Part model, mm, in its own coordinate system. Face numbers are marked on the shaded views. A direction names the side the tool comes from. Coordinates: 2 decimals unless noted, no trailing zeros. Loops run counter-clockwise (first coordinate to the right, second up) from the corner with the lowest first, then second, coordinate; pieces in that order, holes last. Notation, with made-up numbers: M 12.25,70 L 21.25,70 A8 ccw 21.25,77 Z; hole C 61.5,-20.75 d4. An arc over 180 degrees is marked long. Answer as a JSON object with one key per item and string values. Group by question number.
1. Drop flat-ended pins along their axis: pin 1 Ø2 at (x, z) = (21, 4.5) entering from -Y; pin 2 Ø4.5 at (x, y) = (22.5, 27) entering from -Z; pin 3 Ø12 at (x, y) = (25, -12.5) entering from -Z; pin 4 Ø4 at (y, z) = (25.59, -25.5) entering from -X (1 decimal). Give the stop position or say it passes through.
2. Drill centre lines: L1, parallel to Z at x = 37, y = -20.5; L2, parallel to Z at x = 38, y = -22; L3, parallel to Z at x = 3, y = 26. Where is each one in solid material? Low to high.
3. Saw through at B-B on x = 26. Count the separate pieces of the cut face and the enclosed holes in it, then the cut area to 3 significant figures.
4. 3-axis set-ups, long thin cutter, end or side, ignore diameter. For the marked faces 5 and 6: which of +Z, -Z, +X, -X, +Y, -Y reach the whole face in a straight line?
5. Saw through at A-A on y = -19. Write the cut outline in (x, z), then the cut area to 3 significant figures.
6. Mould opens along Z. For the marked faces 1, 2, 3 and 4 say: released by +Z, released by -Z, zero draft, split by the parting line, or undercut.
7. Saw through at C-C on z = -18. Write the cut outline in (x, y).
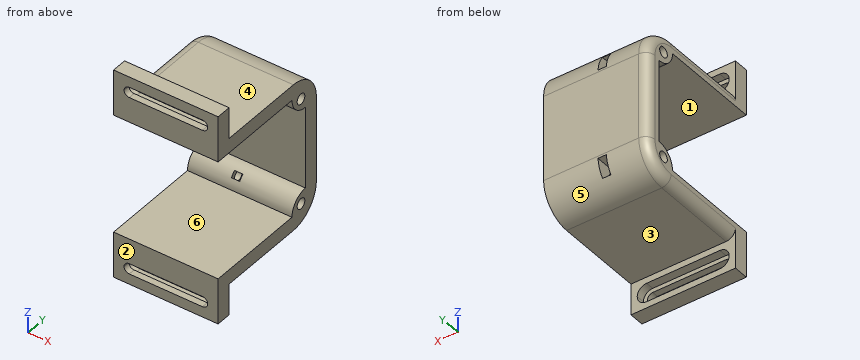
from build123d import *

# Parameters (mm, degrees)
BOSS_EXTRUDE1_DEPTH = 50
SKETCH2_R           = 2.5
CUT_EXTRUDE1_DEPTH  = 50
FILLET1_R           = 15
SKETCH3_W           = 4
SKETCH3_H           = 8
CUT_EXTRUDE2_DEPTH  = 14.54
SKETCH4_W           = 44
SKETCH4_H           = 9
CUT_EXTRUDE3_DEPTH  = 4
SKETCH5_W           = 40
SKETCH5_H           = 5
CUT_EXTRUDE4_DEPTH  = 94.654951818
FILLET2_R           = 2.5
FILLET3_R           = 4.5
FILLET4_R           = 4.5


with BuildPart() as part:
    # Sketch1 → Boss-Extrude1 (new body)
    with BuildSketch(Plane(origin=(0, 0, 0), x_dir=(0, 0, -1), z_dir=(1, 0, 0))):
        with BuildLine():
            Line((35.5, 35.62933491), (-35.5, 35.62933491))
            Line((-35.5, 35.62933491), (-35.5, -21.37066509))
            Line((-35.5, -21.37066509), (-50.5, -21.37066509))
            Line((-50.5, -21.37066509), (-50.5, -28.5))
            Line((-50.5, -28.5), (-28.5, -28.5))
            Line((-28.5, -28.5), (-28.5, 19.7))
            ThreePointArc((-28.5, 19.7), (-22.277460326, 22.277460326), (-19.7, 28.5))
            Line((-19.7, 28.5), (19.7, 28.5))
            ThreePointArc((19.7, 28.5), (22.277460326, 22.277460326), (28.5, 19.7))
            Line((28.5, 19.7), (28.5, -28.5))
            Line((28.5, -28.5), (50.5, -28.5))
            Line((50.5, -28.5), (50.5, -21.37066509))
            Line((50.5, -21.37066509), (35.5, -21.37066509))
            Line((35.5, -21.37066509), (35.5, 35.62933491))
        make_face()
    extrude(amount=BOSS_EXTRUDE1_DEPTH)

    # Sketch2 → Cut-Extrude1 (cut)
    with BuildSketch(Plane.ZY):
        with Locations((-25.5, 25.592902541)):
            Circle(SKETCH2_R)
        with Locations(Location((25.5, 25.592902541, 0), (0, 0, 180))):
            Circle(SKETCH2_R)
    extrude(amount=-CUT_EXTRUDE1_DEPTH, mode=Mode.SUBTRACT)

    # Fillet1
    fillet1_edges = [part.edges().sort_by_distance(p)[0] for p in [
        (25, 35.62933491, 35.5),
        (25, 35.62933491, -35.5),
    ]]
    fillet(fillet1_edges, radius=FILLET1_R)

    # Sketch3 → Cut-Extrude2 (cut)
    with BuildSketch(Plane(origin=(0, 35.62933491, 0), x_dir=(1, 0, 0), z_dir=(0, 1, 0))):
        with Locations((22, 25.5)):
            Rectangle(SKETCH3_W, SKETCH3_H)
        with Locations((22, -25.5)):
            Rectangle(SKETCH3_W, SKETCH3_H)
    extrude(amount=-CUT_EXTRUDE2_DEPTH, mode=Mode.SUBTRACT)

    # Sketch4 → Cut-Extrude3 (cut)
    with BuildSketch(Plane(origin=(0, -21.37066509, 0), x_dir=(1, 0, 0), z_dir=(0, 1, 0))):
        with Locations((25, -43)):
            Rectangle(SKETCH4_W, SKETCH4_H)
        with Locations((25, 43)):
            Rectangle(SKETCH4_W, SKETCH4_H)
    extrude(amount=-CUT_EXTRUDE3_DEPTH, mode=Mode.SUBTRACT)

    # Sketch5 → Cut-Extrude4 (cut, through all)
    with BuildSketch(Plane(origin=(0, -25.37066509, 0), x_dir=(1, 0, 0), z_dir=(0, 1, 0))):
        with Locations((25, -43)):
            Rectangle(SKETCH5_W, SKETCH5_H)
        with Locations((25, 43)):
            Rectangle(SKETCH5_W, SKETCH5_H)
    extrude(amount=-CUT_EXTRUDE4_DEPTH, mode=Mode.SUBTRACT)

    # Fillet2
    fillet2_edges = [part.edges().sort_by_distance(p)[0] for p in [
        (45, -26.935332545, 40.5),
        (45, -26.935332545, 45.5),
        (5, -26.935332545, 45.5),
        (5, -26.935332545, 40.5),
        (5, -26.935332545, -45.5),
        (5, -26.935332545, -40.5),
        (45, -26.935332545, -45.5),
        (45, -26.935332545, -40.5),
    ]]
    fillet(fillet2_edges, radius=FILLET2_R - 0.0001)  # a hair under: the kernel refuses the full size

    # Fillet3
    fillet3_edges = [part.edges().sort_by_distance(p)[0] for p in [
        (3, -23.37066509, 38.5),
        (3, -23.37066509, 47.5),
        (47, -23.37066509, 47.5),
        (47, -23.37066509, 38.5),
        (47, -23.37066509, -47.5),
        (47, -23.37066509, -38.5),
        (3, -23.37066509, -47.5),
        (3, -23.37066509, -38.5),
    ]]
    fillet(fillet3_edges, radius=FILLET3_R - 0.0001)  # a hair under: the kernel refuses the full size

    # Fillet4
    fillet4_edges = [part.edges().sort_by_distance(p)[0] for p in [
        (0, -0.37066509, -35.5),
        (0, -0.37066509, 35.5),
        (0, 35.62933491, 0),
        (0, 31.235936628, -31.106601718),
        (0, 31.235936628, 31.106601718),
    ]]
    fillet(fillet4_edges, radius=FILLET4_R)


solid = part.part
Outcome:
{
 "1": {"pin 1": "stops at y = 28.5", "pin 2": "stops at z = -34.92", "pin 3": "stops at z = -35.5", "pin 4": "passes through"},
 "2": {"L1": "z = -35.5 to -28.5, 28.5 to 35.5", "L2": "z = -50.5 to -47.5, -38.5 to -28.5, 28.5 to 38.5, 47.5 to 50.5", "L3": "z = -34.23 to -27.97, -23.03 to -20.06, 20.06 to 23.03, 27.97 to 34.23"},
 "3": {"separate pieces": "3", "enclosed holes": "2", "area": "1,400 mm²"},
 "4": {"face 5": "-Z, +X, -X, +Y", "face 6": "+X, -X, -Y"},
 "5": {"outline": "M 0,-31 A4.5 ccw 4.5,-35.5 L 50,-35.5 L 50,-28.5 L 0,-28.5 Z; M 0,28.5 L 50,28.5 L 50,35.5 L 4.5,35.5 A4.5 ccw 0,31 Z", "area": "691 mm²"},
 "6": {"face 1": "undercut", "face 2": "zero draft", "face 3": "released by -Z", "face 4": "released by +Z"},
 "7": {"outline": "M 0,28.5 L 50,28.5 L 50,35.63 L 4.5,35.63 A4.5 ccw 0,31.13 Z"}
}
